Work out the finished part from the listing and answer in its coordinate system (mm). A direction names the side the tool comes from. Give positions to 0.01 mm unless a question says otherwise; leave off trailing zeros. Order: outer loops, then holes, each group sorted by start corner. A loop starts at its lowest first (then second) coordinate and runs counter-clockwise, first axis right, second up. Notation, with made-up numbers: (27, 25.25) - (40, 25.25) arc R19 cw to (40, 37.25) - close; hole circle Ø2 at (2.25, 65.5). An arc over 180 degrees is marked (long way). Put each result on its own line as item: value.
```python
from build123d import *

# Parameters (mm, degrees)
IZIM1_R                     = 7
IZIM1_R_2                   = 2.212355073
Y_KSEKLIK_EKSTR_ZYON1_DEPTH = 2
IZIM2_R                     = 3.5
IZIM2_R_2                   = 2.212355073
Y_KSEKLIK_EKSTR_ZYON2_DEPTH = 5
IZIM3_R                     = 1
KES_EKSTR_ZYON1_DEPTH       = 5


with BuildPart() as part:
    # Çizim1 → Yükseklik-Ekstrüzyon1 (new body)
    with BuildSketch(Plane.XY):
        with Locations((-30.711927379, -38.904760786)):
            Circle(IZIM1_R)
        with Locations((-30.711927379, -38.904760786)):
            Circle(IZIM1_R_2, mode=Mode.SUBTRACT)
    extrude(amount=Y_KSEKLIK_EKSTR_ZYON1_DEPTH)

    # Çizim2 → Yükseklik-Ekstrüzyon2 (add)
    with BuildSketch(Plane.XY.offset(2)):
        with Locations((-30.711927379, -38.904760786)):
            Circle(IZIM2_R)
        with Locations((-30.711927379, -38.904760786)):
            Circle(IZIM2_R_2, mode=Mode.SUBTRACT)
    extrude(amount=-Y_KSEKLIK_EKSTR_ZYON2_DEPTH)

    # Çizim3 → Kes-Ekstrüzyon1 (cut)
    with BuildSketch(Plane(origin=(0, 0, 0), x_dir=(-1, 0, 0), z_dir=(0, 0, -1))):
        with Locations((30.711927379, -34.154760786)):
            Circle(IZIM3_R)
        with Locations((34.825548047, -41.279760786)):
            Circle(IZIM3_R)
        with Locations((26.598306711, -41.279760786)):
            Circle(IZIM3_R)
    extrude(amount=-KES_EKSTR_ZYON1_DEPTH, mode=Mode.SUBTRACT)


solid = part.part
```
(1) A tool of negligible diameter and unlimited length cuts with its end or side. For faces 1 (the face through (-29.918, -34.763, 0.986)), 2 (the face through (-34, -37, 0)), from which of +Z, -Z, +X, -X, +Y, -Y can it reach the whole face along a straight path? Write none if from no direction.
Geometry check:
face 1: +Z, -Z
face 2: -Z
(2) Section D-D, the plane y = -40.5 is taken. Write down the section's boundary in (x, z), then the cut area to 3 significant figures.
Geometry check:
outline: (-37.53, 0) - (-35.45, 0) - (-35.45, 2) - (-37.53, 2) - close; (-34.2, 0) - (-33.83, 0) - (-33.83, -3) - (-32.24, -3) - (-32.24, 2) - (-34.2, 2) - close; (-29.18, -3) - (-27.6, -3) - (-27.6, 0) - (-27.22, 0) - (-27.22, 2) - (-29.18, 2) - close; (-25.97, 0) - (-23.9, 0) - (-23.9, 2) - (-25.97, 2) - close
area: 25.6 mm²
(3) Given pin 1 (2.5 mm diameter, centred on x = -30.71, y = -34.15, fed in from +Z); pin 2 (2 mm diameter, centred on x = -33.5, z = 0, fed in from +Y), each flat-ended and moving along its own axis, determine where each tip first touches the part or whether it passes through.
Geometry check:
pin 1: stops at z = 2
pin 2: stops at y = -32.14
(4) Section C-C, the plane z = 1.05 is taken. Write down the section's boundary in (x, y).
Geometry check:
outline: circle Ø14 at (-30.71, -38.9); hole circle Ø2 at (-34.83, -41.28); hole circle Ø4.42 at (-30.71, -38.9); hole circle Ø2 at (-30.71, -34.15); hole circle Ø2 at (-26.6, -41.28)
(5) Section A-A, the plane x = -29 is taken. Write down the section's boundary in (y, z), then the cut area to 3 significant figures.
Geometry check:
outline: (-45.69, 0) - (-41.96, 0) - (-41.96, -3) - (-40.31, -3) - (-40.31, 2) - (-45.69, 2) - close; (-37.5, -3) - (-35.85, -3) - (-35.85, 0) - (-32.12, 0) - (-32.12, 2) - (-37.5, 2) - close
area: 31.5 mm²
(6) Section B-B, the plane y = -34.5 is taken. Write down the section's boundary in (x, z).
Geometry check:
outline: (-36.15, 0) - (-31.65, 0) - (-31.65, 2) - (-36.15, 2) - close; (-29.77, 0) - (-25.27, 0) - (-25.27, 2) - (-29.77, 2) - close
(7) Determine the mould class of faces 3 (the face through (-37.705, -38.597, 0.986)), 4 (the face through (-34.609, -42.256, 0.986)), 5 (the face through (-28, -39, -3)) for opening direction X: pulls with the +X half, pulls with the -X half, needs draft (parallel to the pull), parting line crosses it, or undercut.
Geometry check:
face 3: parting line crosses it
face 4: undercut
face 5: needs draft
(8) Straight lines are drawn through the part: line 1 (Y direction, x = -31.5, z = 1.4); line 2 (Z direction, x = -34.5, y = -37.75); line 3 (X direction, y = -39, z = 1.75). For each, find the intervals that lie inside material, in ascending order.
Geometry check:
line 1: y = -45.86 to -40.97, -36.84 to -34.77, -33.54 to -31.95
line 2: z = 0 to 2
line 3: x = -37.71 to -32.92, -28.5 to -23.71
